from build123d import *

# Parameters (mm, degrees)
SKETCH1_W              = 622.3
SKETCH1_H              = 787.4
BOSS_EXTRUDE1_DEPTH    = 19.05
SKETCH2_W              = 88.9
SKETCH2_H              = 38.1
CUT_EXTRUDE1_DEPTH     = 1004.802247706
F_10_CLEARANCE_HOLE6_D = 5.6134


with BuildPart() as part:
    # Sketch1 → Boss-Extrude1 (new body)
    with BuildSketch(Plane(origin=(0, 0, 0), x_dir=(0, 0, -1), z_dir=(1, 0, 0))):
        with Locations((-311.15, 393.7)):
            Rectangle(SKETCH1_W, SKETCH1_H)
    extrude(amount=-BOSS_EXTRUDE1_DEPTH)

    # Sketch2 → Cut-Extrude1 (cut, through all)
    with BuildSketch(Plane.ZY.offset(19.05)):
        with Locations((44.45, 768.35)):
            Rectangle(SKETCH2_W, SKETCH2_H)
        with Locations((577.85, 768.35)):
            Rectangle(SKETCH2_W, SKETCH2_H)
        with Locations((577.85, 19.05)):
            Rectangle(SKETCH2_W, SKETCH2_H)
        with Locations((44.45, 19.05)):
            Rectangle(SKETCH2_W, SKETCH2_H)
    extrude(amount=-CUT_EXTRUDE1_DEPTH, mode=Mode.SUBTRACT)

    # #10 Clearance Hole6 (through all)
    with Locations(Plane(origin=(0, 0, 0), x_dir=(0, 0, -1), z_dir=(1, 0, 0))):
        with Locations((-603.25, 50.8), (-603.25, 63.5), (-19.05, 50.8), (-19.05, 63.5), (-19.05, 723.9), (-19.05, 736.6), (-603.25, 723.9), (-603.25, 736.6)):
            Hole(F_10_CLEARANCE_HOLE6_D / 2)


solid = part.part
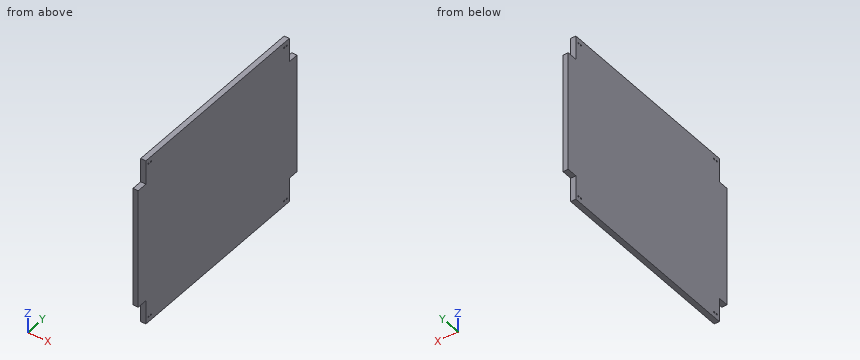
Verification items for the finished model (mm, model axes). Give positions to 0.01 mm unless a question says otherwise; leave off trailing zeros. Write each loop counter-clockwise with the first axis right and the second up, starting at its lowest first coordinate (ties: lowest second). Pieces come first, ordered by that corner, then holes. Notation, with made-up numbers: (7, 88) - (54, 88) arc R20 cw to (54, 113) - close; hole circle Ø6 at (-24, 59.5). An arc over 180 degrees is marked (long way). Answer as CSV lines item,"result". Start each with the question number.
1. Depth check by flat-ended pin: pin 1 (9.5 mm diameter, centred on x = -5.5, y = 18, fed in from +Z); pin 2 (9.5 mm diameter, centred on x = -12.5, y = 774, fed in from -Z); pin 3 (9.5 mm diameter, centred on x = -7.5, z = 594, fed in from +Y). Enter the tip coordinate at first touch or a pass-through.
2. Sectioned sample at A-A (x = -4.25). Count the separate pieces of the cut face and the enclosed holes in it, then the cut area to 3 significant figures.
3. Thickness scan on line 1 (Z direction, x = -6.5, y = 736.6); line 2 (Y direction, x = -9, z = 19.05); line 3 (Y direction, x = -6, z = 591.5). Record the ranges inside material, lowest first.
4. Sectioned sample at B-B (z = 45.5). Record the boundary of the cut face in (x, y), then the cut area to 3 significant figures.
Derived:
1,pin 1,"z = 533.4"
1,pin 2,"z = 88.9"
1,pin 3,"y = 749.3"
2,separate pieces,"1"
2,enclosed holes,"8"
2,area,"476,000 mm²"
3,line 1,"0 to 16.24, 21.86 to 600.44, 606.06 to 622.3"
3,line 2,"38.1 to 47.99, 53.61 to 60.69, 66.31 to 721.09, 726.71 to 733.79, 739.41 to 749.3"
3,line 3,"38.1 to 749.3"
4,outline,"(-19.05, 38.1) - (0, 38.1) - (0, 749.3) - (-19.05, 749.3) - close"
4,area,"13,500 mm²"
